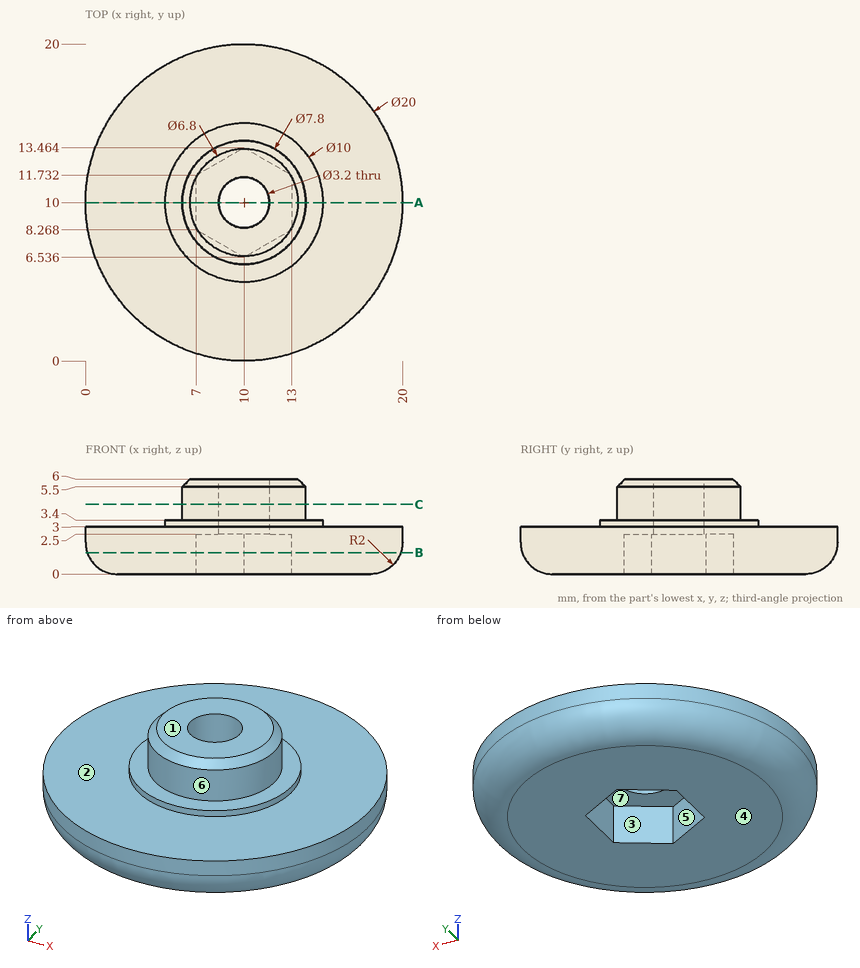
Answer from the drawing. Dimensions are ordinates in mm from the lowest x, y and z of the part. A direction names the side the tool comes from. Give positions to 0.01 mm unless a question says otherwise; leave off trailing zeros. Order: outer loops, then holes, each group sorted by start corner. A loop starts at its lowest first (then second) coordinate and runs counter-clockwise, first axis right, second up. Notation, with made-up numbers: (-21.75, 62) - (-2.75, 62) arc R31 cw to (-2.75, 96) - close; hole circle Ø7 at (19.25, 71.5). An arc over 180 degrees is marked (long way). Use one line per item in the form item = value.
1) Each of these flat-tipped pins is pushed along its axis until it touches: pin 1 (0.8 mm diameter, centred on y = 10, z = 1, fed in from +X); pin 2 (11 mm diameter, centred on x = 9.5, y = 9, fed in from +Z); pin 3 (1 mm diameter, centred on x = 2.5, y = 16, fed in from -Z); pin 4 (1.2 mm diameter, centred on y = 10.5, z = 0.5, fed in from -X). Where does it stop, or does it pass through?
Verdict:
pin_1 = 19.91
pin_2 = 6
pin_3 = 0.33
pin_4 = 0.23
2) Find section B-B on z = 1.35. Determine the outline of the cut face in (x, y).
Verdict:
outline = circle Ø19.78 at (10, 10); hole (7, 8.27) - (10, 6.54) - (13, 8.27) - (13, 11.73) - (10, 13.46) - (7, 11.73) - close
3) Find section C-C on z = 4.4. Determine the outline of the cut face in (x, y), and give its area (3 significant figures).
Verdict:
outline = circle Ø7.8 at (10, 10); hole circle Ø3.2 at (10, 10)
area = 39.7 mm^2
4) Find section A-A on y = 10. Determine the outline of the cut face in (x, z).
Verdict:
outline = (0, 2) arc R2 ccw to (2, 0) - (7, 0) - (7, 2.5) - (8.4, 2.5) - (8.4, 6) - (6.6, 6) - (6.1, 5.5) - (6.1, 3.4) - (5, 3.4) - (5, 3) - (0, 3) - close; (11.6, 2.5) - (13, 2.5) - (13, 0) - (18, 0) arc R2 ccw to (20, 2) - (20, 3) - (15, 3) - (15, 3.4) - (13.9, 3.4) - (13.9, 5.5) - (13.4, 6) - (11.6, 6) - close
5) Consider probe 1 along X at (y, z) = (10, 4.9); probe 2 along Z at (x, y) = (2.5, 13). Determine where each line is inside the solid, lowest interval first. Write a range as [from, to].
Verdict:
probe_1 = [6.1, 8.4], [11.6, 13.9]
probe_2 = [0, 3]
6) The mould has two halves that part along X. Classify the marked faces 4, 5, 6 and 7: released by +X, released by -X, zero draft, split by the parting line, or undercut.
Verdict:
face_4 = zero draft
face_5 = undercut
face_6 = split by the parting line
face_7 = undercut
7) For the marked faces 1, 2 and 3, determine the directions among +Z, -Z, +X, -X, +Y, -Y from which every point of the face is accessible in a straight line to the end or side of a thin tool.
Verdict:
face_1 = +Z, +X, -X, +Y, -Y
face_2 = +Z
face_3 = -Z
